Design review of the part built by this model. Coordinates are the model's own, in mm. Round coordinates to 2 decimals unless told otherwise and drop trailing zeros. Order: outer loops, then holes, each group sorted by start corner. A loop starts at its lowest first (then second) coordinate and runs counter-clockwise, first axis right, second up. Notation, with made-up numbers: (50.5, 12) - (102.5, 12) arc R31 ccw to (102.5, 41) - close; hole circle Ø2 at (85, 28). An arc over 180 degrees is marked (long way). Use CSV: the item, a comma, the result in double quotes.
from build123d import *

# Parameters (mm, degrees)
F0_W     = 19.05
F0_H     = 152.4
F0_W_2   = 152.4
F0_H_2   = 19.05
F1_DEPTH = 19.05


with BuildPart() as f1:
    # F0 (on Top) → F1 (new body)
    with BuildSketch(Plane.XY):
        Polygon((-441.325, 0), (-720.725, 0), (-720.725, -88.9), (-720.725, -241.3), (-720.725, -342.9), (720.725, -342.9), (720.725, -241.3), (720.725, -88.9), (720.725, 0), (441.325, 0), (288.925, 0), (-288.925, 0), align=None)
        with Locations((-243.416667, -165.1)):
            Rectangle(F0_W, F0_H, mode=Mode.SUBTRACT)
        with Locations((243.416667, -165.1)):
            Rectangle(F0_W, F0_H, mode=Mode.SUBTRACT)
        with Locations((-365.125, 9.525)):
            Rectangle(F0_W_2, F0_H_2)
        with Locations((365.125, 9.525)):
            Rectangle(F0_W_2, F0_H_2)
        with Locations((730.25, -165.1)):
            Rectangle(F0_W, F0_H)
        with Locations((-730.25, -165.1)):
            Rectangle(F0_W, F0_H)
    extrude(amount=F1_DEPTH)


solid = f1.part
1) Insertion check: pin 1 Ø9.5 at (y, z) = (7.5, 12.5) entering from +X (3 decimals); pin 2 Ø5.5 at (x, z) = (577, 12) entering from +Y; pin 3 Ø5.5 at (y, z) = (-271, 7.5) entering from -X (3 decimals). Each pin has a flat end and moves straight along its axis. Give the tip position at first contact, or say it passes through.
Data:
pin 1,"stops at x = 441.325"
pin 2,"stops at y = 0"
pin 3,"stops at x = -720.725"
2) We need section D-D (y = -18.5). Give the boundary of the cut face in (x, z) (3 decimals), then the cut area to 3 significant figures.
Data:
outline,"(-720.725, 0) - (720.725, 0) - (720.725, 19.05) - (-720.725, 19.05) - close"
area,"27,500 mm2"
3) To check wall thickness, follow L1, parallel to X at y = -113.5, z = 2 (3 decimals); L2, parallel to X at y = -271, z = 14.5 (3 decimals); L3, parallel to Y at x = 276, z = 14. State the ranges of each line that lie inside material, in increasing order. Write a range as from..to.
Data:
L1,"x = -739.775..-252.942, -233.892..233.892, 252.942..739.775"
L2,"x = -720.725..720.725"
L3,"y = -342.9..0"
4) We need section C-C (x = 151.5). Give the boundary of the cut face in (y, z), then the cut area to 3 significant figures.
Data:
outline,"(-342.9, 0) - (0, 0) - (0, 19.05) - (-342.9, 19.05) - close"
area,"6,530 mm2"
5) We need section A-A (y = -107.5). Give the boundary of the cut face in (x, z) (3 decimals), then the cut area to 3 significant figures.
Data:
outline,"(-739.775, 0) - (-252.942, 0) - (-252.942, 19.05) - (-739.775, 19.05) - close; (-233.892, 0) - (233.892, 0) - (233.892, 19.05) - (-233.892, 19.05) - close; (252.942, 0) - (739.775, 0) - (739.775, 19.05) - (252.942, 19.05) - close"
area,"27,500 mm2"
6) We need section B-B (z = 7). Give the boundary of the cut face in (x, y) (3 decimals), then the cut area to 3 significant figures.
Data:
outline,"(-739.775, -241.3) - (-720.725, -241.3) - (-720.725, -342.9) - (720.725, -342.9) - (720.725, -241.3) - (739.775, -241.3) - (739.775, -88.9) - (720.725, -88.9) - (720.725, 0) - (441.325, 0) - (441.325, 19.05) - (288.925, 19.05) - (288.925, 0) - (-288.925, 0) - (-288.925, 19.05) - (-441.325, 19.05) - (-441.325, 0) - (-720.725, 0) - (-720.725, -88.9) - (-739.775, -88.9) - close; hole (-252.942, -241.3) - (-233.892, -241.3) - (-233.892, -88.9) - (-252.942, -88.9) - close; hole (233.892, -241.3) - (252.942, -241.3) - (252.942, -88.9) - (233.892, -88.9) - close"
area,"500,000 mm2"
